CAD build for the part. Positions are in the model's coordinates, mm. A direction names the side the tool comes from. Give positions to 0.01 mm unless a question says otherwise; leave off trailing zeros. Loops run counter-clockwise (first coordinate to the right, second up) from the corner with the lowest first, then second, coordinate; pieces in that order, holes last. Notation, with made-up numbers: (36, -9.5) - (86, -9.5) arc R24 cw to (86, 22.5) - close; hole circle Ø2 at (-22.75, 86). An arc over 180 degrees is marked (long way). Return JSON: item names as keys, results as strings.
from build123d import *

# Parameters (mm, degrees)
SKETCH2_W               = 30.5
SKETCH2_H               = 10.5
BOSS_EXTRUDE1_DEPTH     = 4
FILLET1_R               = 5
SKETCH3_R               = 2.4
BOSS_EXTRUDE2_DEPTH     = 10
CUT_EXTRUDE1_DEPTH      = 148.39402973
CUT_EXTRUDE1_DEPTH_BACK = 148.39402973
SKETCH4_R               = 1.4
SKETCH4_R_2             = 1.1
CUT_EXTRUDE2_DEPTH      = 148.719328458
CUT_EXTRUDE2_DEPTH_BACK = 148.719328458
SKETCH5_R               = 1.4
FILLET2_R               = 3
FILLET3_R               = 3
FILLET4_R               = 3


with BuildPart() as part:
    # Sketch2 → Boss-Extrude1 (new body)
    with BuildSketch(Plane(origin=(0, 0, 0), x_dir=(1, 0, 0), z_dir=(0, 1, 0))):
        with BuildLine():
            Line((-120, 50), (-85, 50))
            ThreePointArc((-85, 50), (-77.5, 42.5), (-85, 35))
            Line((-85, 35), (-85, 0))
            Line((-85, 0), (0, 0))
            Line((0, 0), (0, 85))
            Line((0, 85), (-120, 85))
            Line((-120, 85), (-120, 50))
        make_face()
        with Locations((-100.25, 69.75)):
            Rectangle(SKETCH2_W, SKETCH2_H, mode=Mode.SUBTRACT)
    extrude(amount=BOSS_EXTRUDE1_DEPTH)

    # Fillet1
    fillet1_edges = [part.edges().sort_by_distance(p)[0] for p in [
        (0, 2, 0),
        (-85, 2, 0),
        (-85, 2, -35),
        (-120, 2, -50),
        (-120, 2, -85),
        (0, 2, -85),
    ]]
    fillet(fillet1_edges, radius=FILLET1_R)

    # Sketch3 → Boss-Extrude2 (add)
    with BuildSketch(Plane(origin=(0, 4, 0), x_dir=(1, 0, 0), z_dir=(0, 1, 0))):
        with Locations(Location((-6.586230152, 80.5, 0), (0, 0, 90))):
            Circle(SKETCH3_R)
        with Locations(Location((-40.786230152, 80.5, 0), (0, 0, 90))):
            Circle(SKETCH3_R)
        with Locations(Location((-40.786230152, 5.300086959, 0), (0, 0, 90))):
            Circle(SKETCH3_R)
        with Locations(Location((-6.586230152, 5.3, 0), (0, 0, 90))):
            Circle(SKETCH3_R)
    extrude(amount=BOSS_EXTRUDE2_DEPTH)

    # Sketch4 → Cut-Extrude1 (cut, two sides: drawn at the far end of the back side and taken through both)
    with BuildSketch(Plane(origin=(0, 4, 0), x_dir=(1, 0, 0), z_dir=(0, 1, 0)).offset(-CUT_EXTRUDE1_DEPTH_BACK)):
        with Locations(Location((-8.5, 50, 0), (0, 0, 270))):
            Circle(SKETCH4_R)
        with Locations(Location((-8.5, 35.2, 0), (0, 0, 270))):
            Circle(SKETCH4_R)
        with Locations(Location((-8, 15, 0), (0, 0, 270))):
            Circle(SKETCH4_R_2)
        with Locations(Location((-22, 6.4, 0), (0, 0, 270))):
            Circle(SKETCH4_R)
        with Locations(Location((-22, 77.4, 0), (0, 0, 270))):
            Circle(SKETCH4_R)
        with Locations(Location((-10.315869942, 72.297665639, 0), (0, 0, 270))):
            Circle(SKETCH4_R_2)
    extrude(amount=CUT_EXTRUDE1_DEPTH + CUT_EXTRUDE1_DEPTH_BACK, mode=Mode.SUBTRACT)

    # Sketch5 → Cut-Extrude2 (cut, two sides: drawn at the far end of the back side and taken through both)
    with BuildSketch(Plane.XZ.offset(-CUT_EXTRUDE2_DEPTH_BACK)):
        with Locations(Location((-32.695307694, -77.13410082, 0), (0, 0, 270))):
            Circle(SKETCH5_R)
        with Locations(Location((-73.795307694, -77.13410082, 0), (0, 0, 270))):
            Circle(SKETCH5_R)
        with Locations(Location((-77.058410355, -11.13410082, 0), (0, 0, 270))):
            Circle(SKETCH5_R)
        with Locations(Location((-29.058410355, -11.13410082, 0), (0, 0, 270))):
            Circle(SKETCH5_R)
    extrude(amount=CUT_EXTRUDE2_DEPTH + CUT_EXTRUDE2_DEPTH_BACK, mode=Mode.SUBTRACT)

    # Fillet2
    fillet2_edges = [part.edges().sort_by_distance(p)[0] for p in [
        (-6.586230152, 4, -2.9),
    ]]
    fillet(fillet2_edges, radius=FILLET2_R)

    # Fillet3
    fillet3_edges = [part.edges().sort_by_distance(p)[0] for p in [
        (-40.786230152, 4, -2.900086959),
    ]]
    fillet(fillet3_edges, radius=FILLET3_R)

    # Fillet4
    fillet4_edges = [part.edges().sort_by_distance(p)[0] for p in [
        (-6.586230152, 4, -78.1),
        (-40.786230152, 4, -78.1),
    ]]
    fillet(fillet4_edges, radius=FILLET4_R)


solid = part.part
1. Cut at A-A, the plane y = 11.5. Write the cut outline in (x, z), plus the area to 3 significant figures.
Values follow:
{"outline": "circle Ø4.8 at (-40.79, -80.5); circle Ø4.8 at (-40.79, -5.3); circle Ø4.8 at (-6.59, -80.5); circle Ø4.8 at (-6.59, -5.3)", "area": "72.4 mm²"}
2. Which spindle directions (+Z, -Z, +X, -X, +Y, -Y) get a long thin tool onto all of the face, cutting with end or side? Do faces 4 (the face through (-84.16, 2.03, -33.82)), 5 (the face through (-100, 2, -50)), 6 (the face through (-115.5, 2, -70)), 7 (the face through (-5.67, 10.38, -82.72)). Say none if no direction does.
Values follow:
{"face 4": "-X, +Y, -Y", "face 5": "+Z, -X, +Y, -Y", "face 6": "+Y, -Y", "face 7": "+Y"}
3. Pull direction X, two halves, no side cores. Call faces 1 (the face through (-85, 2, -18)), 2 (the face through (-23.24, 1.97, -5.75)), 3 (the face through (0, 2, -42)): +X half, -X half, draft (parallel to the pull), parting line (faces both ways), or undercut.
Values follow:
{"face 1": "-X half", "face 2": "undercut", "face 3": "+X half"}
4. Drop flat-ended pins along their axis: P1, Ø10, axis at x = -99, z = -58.5, coming from the +Y side; P2, Ø2, axis at x = -102.5, y = 2.5, coming from the +Z side; P3, Ø4.5, axis at y = 1.5, z = -12, coming from the -X side. Give the stop position or say it passes through.
Values follow:
{"P1": "stops at y = 4", "P2": "stops at z = -50", "P3": "stops at x = -85"}
5. Drill centre lines: probe 1 along Z at (x, y) = (-22, 1.8); probe 2 along Z at (x, y) = (-8, 2.3); probe 3 along Z at (x, y) = (-8.5, 2.9). Where is each one in solid material? Low to high.
Values follow:
{"probe 1": "z = -85 to -78.8, -76 to -7.8, -5 to 0", "probe 2": "z = -85 to -51.31, -48.69 to -36.51, -33.89 to -16.1, -13.9 to 0", "probe 3": "z = -85 to -51.4, -48.6 to -36.6, -33.8 to -15.98, -14.02 to 0"}
